Autodesk Inventor part; units mm, degrees
ref_plane "YZ Plane" through (0, 0, 0) normal (1, 0, 0) x (0, 1, 0)
ref_plane "XZ Plane" through (0, 0, 0) normal (0, 1, 0) x (-1, 0, 0)
ref_plane "XY Plane" through (0, 0, 0) normal (0, 0, 1) x (1, 0, 0)
sketch "Sketch1" plane through (0, 0, 0) normal (0, 1, 0) x (-1, 0, 0)
  line L0 (0, 6.4) -> (0.794, 6.4)
  line L1 (0, 6.4) -> (-0.794, 6.4)
  line L2 (0.794, 6.4) -> (0.794, 12.6752)
  line L3 (-0.794, 6.4) -> (-0.794, 12.6752)
  line L4 (3.7618, 5.1777) -> (4.4042, 4.711)
  line L5 (3.7618, 5.1777) -> (3.1195, 5.6444)
  line L6 (4.4042, 4.711) -> (8.0926, 9.7877)
  line L7 (3.1195, 5.6444) -> (6.8079, 10.7211)
  line L8 (6.0868, 1.9777) -> (6.3321, 1.2226)
  line L9 (6.0868, 1.9777) -> (5.8414, 2.7328)
  line L10 (6.3321, 1.2226) -> (12.3001, 3.1617)
  line L11 (5.8414, 2.7328) -> (11.8094, 4.672)
  line L12 (6.0868, -1.9777) -> (5.8414, -2.7328)
  line L13 (6.0868, -1.9777) -> (6.3321, -1.2226)
  line L14 (5.8414, -2.7328) -> (11.8094, -4.672)
  line L15 (6.3321, -1.2226) -> (12.3001, -3.1617)
  line L16 (3.7618, -5.1777) -> (3.1195, -5.6444)
  line L17 (3.7618, -5.1777) -> (4.4042, -4.711)
  line L18 (3.1195, -5.6444) -> (6.8079, -10.7211)
  line L19 (4.4042, -4.711) -> (8.0926, -9.7877)
  line L20 (0, -6.4) -> (-0.794, -6.4)
  line L21 (0, -6.4) -> (0.794, -6.4)
  line L22 (-0.794, -6.4) -> (-0.794, -12.6752)
  line L23 (0.794, -6.4) -> (0.794, -12.6752)
  line L24 (-3.7618, -5.1777) -> (-4.4042, -4.711)
  line L25 (-3.7618, -5.1777) -> (-3.1195, -5.6444)
  line L26 (-4.4042, -4.711) -> (-8.0926, -9.7877)
  line L27 (-3.1195, -5.6444) -> (-6.8079, -10.7211)
  line L28 (-6.0868, -1.9777) -> (-6.3321, -1.2226)
  line L29 (-6.0868, -1.9777) -> (-5.8414, -2.7328)
  line L30 (-6.3321, -1.2226) -> (-12.3001, -3.1617)
  line L31 (-5.8414, -2.7328) -> (-11.8094, -4.672)
  line L32 (-6.0868, 1.9777) -> (-5.8414, 2.7328)
  line L33 (-6.0868, 1.9777) -> (-6.3321, 1.2226)
  line L34 (-5.8414, 2.7328) -> (-11.8094, 4.672)
  line L35 (-6.3321, 1.2226) -> (-12.3001, 3.1617)
  line L36 (-3.7618, 5.1777) -> (-3.1195, 5.6444)
  line L37 (-3.7618, 5.1777) -> (-4.4042, 4.711)
  line L38 (-3.1195, 5.6444) -> (-6.8079, 10.7211)
  line L39 (-4.4042, 4.711) -> (-8.0926, 9.7877)
  arc A0 (6.8079, 10.7211) -> (0.794, 12.6752) centre (0, 0) ccw
  arc A1 (-0.794, 12.6752) -> (-6.8079, 10.7211) centre (0, 0) ccw
  arc A2 (-8.0926, 9.7877) -> (-11.8094, 4.672) centre (0, 0) ccw
  arc A3 (-12.3001, 3.1617) -> (-12.3001, -3.1617) centre (0, 0) ccw
  arc A4 (-11.8094, -4.672) -> (-8.0926, -9.7877) centre (0, 0) ccw
  arc A5 (-6.8079, -10.7211) -> (-0.794, -12.6752) centre (0, 0) ccw
  arc A6 (0.794, -12.6752) -> (6.8079, -10.7211) centre (0, 0) ccw
  arc A7 (8.0926, -9.7877) -> (11.8094, -4.672) centre (0, 0) ccw
  arc A8 (12.3001, -3.1617) -> (12.3001, 3.1617) centre (0, 0) ccw
  arc A9 (11.8094, 4.672) -> (8.0926, 9.7877) centre (0, 0) ccw
  circle A10 centre (0, 0) radius 3.175
  dimension "d1" = 0.794
  dimension "d2" = 0.794
  dimension "d3" = 6.4
  dimension "d6" = 360
  dimension "d8" = 12.7
  dimension "d9" = 6.35
extrude "Extrusion1" add sketch "Sketch1" along normal blind 1.556
properties part number "HeatSinkWasher"
Here's how the part is built. I have some questions about the finished solid (model axes, mm). A direction names the side the tool comes from. Round coordinates to 2 decimals unless told otherwise and drop trailing zeros. Write each loop counter-clockwise with the first axis right and the second up, starting at its lowest first coordinate (ties: lowest second). Pieces come first, ordered by that corner, then holes.
Q1. If we section it at B-B on x = 7.75: Write out the boundary of the cut face in (y, z).
Q2. If we mould it in two halves opening along Z, with no side actions, what happens to faces 1 (the flat face through (0, 1, -6.4)), 2 (the flat face through (0.794, 1, -9)), 3 (the flat face through (0, 1, 6.4)), 4 (the flat face through (4.94, 0.77, -8.15))? For each: +Z half, -Z half, draft (parallel to the pull), parting line (faces both ways), or undercut.
Q3. If we section it at D-D on z = -9: Write out the boundary of the cut face in (x, y).
Q4. If we section it at C-C on x = 0: Write out the boundary of the cut face in (y, z) (3 decimals), plus the area to 3 significant figures.
Q5. Will these pins go through, and if not, where does the flat tip stop? P1, Ø0.8, axis at y = 0.5, z = -8.5, coming from the +X side; P2, Ø0.8, axis at x = 0, y = 0.5, coming from the +Z side.
Q6. Which directions (+Z, -Z, +X, -X, +Y, -Y) give clear straight access to the entire face, cutting with the end or side of a thin tool? Please do faces 5 (the flat face through (-9.274, 0.767, 2.179)), 6 (the flat face through (-0.794, 1, -9)), 7 (the flat face through (-3, 0, -3)).
Q7. Please list where these lines run through material, in increasing order: probe 1 along Z at (x, y) = (0, 0.8) (3 decimals); probe 2 along Z at (x, y) = (-8, 0.9); probe 3 along Z at (x, y) = (-7.25, 0.9).
Q8. If we section it at A-A on z = 0: Write out the boundary of the cut face in (x, y) (3 decimals), plus the area to 3 significant figures.
Answer below:
1. outline: (0, -9.32) - (1.56, -9.32) - (1.56, -3.35) - (0, -3.35) - close; (0, -1.68) - (1.56, -1.68) - (1.56, 1.68) - (0, 1.68) - close; (0, 3.35) - (1.56, 3.35) - (1.56, 9.32) - (0, 9.32) - close
2. face 1: -Z half
2. face 2: draft
2. face 3: +Z half
2. face 4: undercut
3. outline: (-8.96, 0) - (-7.52, 0) - (-7.52, 1.56) - (-8.96, 1.56) - close; (-5.56, 0) - (-0.79, 0) - (-0.79, 1.56) - (-5.56, 1.56) - close; (0.79, 0) - (5.56, 0) - (5.56, 1.56) - (0.79, 1.56) - close; (7.52, 0) - (8.96, 0) - (8.96, 1.56) - (7.52, 1.56) - close
4. outline: (0, -6.4) - (1.556, -6.4) - (1.556, -3.175) - (0, -3.175) - close; (0, 3.175) - (1.556, 3.175) - (1.556, 6.4) - (0, 6.4) - close
4. area: 10.0 mm2
5. P1: stops at x = 9.78
5. P2: stops at z = 6.4
6. face 5: +Y, -Y
6. face 6: -Z, +Y, -Y
6. face 7: +Z, -Z, +X, -X, -Y
7. probe 1: z = -6.4 to -3.175, 3.175 to 6.4
7. probe 2: z = -9.66 to -3.43, -1.76 to 1.76, 3.43 to 9.66
7. probe 3: z = -8.63 to -3.19, -1.52 to 1.52, 3.19 to 8.63
8. outline: (-12.7, 0) - (-3.175, 0) - (-3.175, 1.556) - (-12.7, 1.556) - close; (3.175, 0) - (12.7, 0) - (12.7, 1.556) - (3.175, 1.556) - close
8. area: 29.6 mm2
